Source: CAD feature listing. Evaluate the final solid. Frame: model axes, mm. Coordinates: 2 decimals unless noted, no trailing zeros. Order: outer loops, then holes, each group sorted by start corner. A loop starts at its lowest first (then second) coordinate and runs counter-clockwise, first axis right, second up. Notation, with made-up numbers: (43.5, -11.5) -> (76.5, -11.5) arc R30 cw to (76.5, 20.5) -> close; hole circle Ø5 at (75.25, 14.5). An arc over 180 degrees is marked (long way). Put each result on its own line as item: value.
from build123d import *

# Parameters (mm, degrees)
F1_DEPTH = 2
F2_R     = 5
F4_DEPTH = 2
F6_DEPTH = 2


# Not quite as in the source:
# - a feature names something its author has since deleted; it is built from what else it names


with BuildPart() as f1:
    # F0 (on Front) → F1 (new body)
    with BuildSketch(Plane.XZ):
        with BuildLine():
            Line((0, 5.5), (0, 0))
            Line((0, 0), (40, 0))
            Line((40, 0), (40, 5.5))
            Line((40, 5.5), (25, 5.5))
            ThreePointArc((25, 5.5), (22, 2.5), (19, 5.5))
            Line((19, 5.5), (0, 5.5))
        make_face()
        with BuildLine():
            Line((40, 5.5), (40, 0))
            Line((40, 0), (40, -2.5))
            ThreePointArc((40, -2.5), (41.05572809, 1.972135955), (44, 5.5))
            Line((44, 5.5), (40, 5.5))
        make_face()
        with BuildLine():
            Line((0, 11), (0, 5.5))
            Line((0, 5.5), (19, 5.5))
            ThreePointArc((19, 5.5), (22, 8.5), (25, 5.5))
            Line((25, 5.5), (40, 5.5))
            Line((40, 5.5), (40, 11))
            Line((40, 11), (0, 11))
        make_face()
        with BuildLine():
            Line((40, 11), (40, 5.5))
            Line((40, 5.5), (44, 5.5))
            ThreePointArc((44, 5.5), (41.05572809, 9.027864045), (40, 13.5))
            Line((40, 13.5), (40, 11))
        make_face()
        with BuildLine():
            Line((45, -2.5), (40, -2.5))
            ThreePointArc((40, -2.5), (50, -12.5), (60, -2.5))
            ThreePointArc((60, -2.5), (58.94427191, 1.972135955), (56, 5.5))
            ThreePointArc((56, 5.5), (53.1622776602, 4.0131670195), (50, 3.5))
            Line((50, 3.5), (50, 2.5))
            ThreePointArc((50, 2.5), (53.5355339059, 1.0355339059), (55, -2.5))
            ThreePointArc((55, -2.5), (50, -7.5), (45, -2.5))
        make_face()
        with BuildLine():
            ThreePointArc((44, 5.5), (41.05572809, 1.972135955), (40, -2.5))
            Line((40, -2.5), (45, -2.5))
            ThreePointArc((45, -2.5), (46.4644660941, 1.0355339059), (50, 2.5))
            Line((50, 2.5), (50, 3.5))
            ThreePointArc((50, 3.5), (46.8377223398, 4.0131670195), (44, 5.5))
        make_face()
        with BuildLine():
            ThreePointArc((40, 13.5), (41.05572809, 9.027864045), (44, 5.5))
            ThreePointArc((44, 5.5), (46.8377223398, 6.9868329805), (50, 7.5))
            Line((50, 7.5), (50, 8.5))
            ThreePointArc((50, 8.5), (46.4644660941, 9.9644660941), (45, 13.5))
            Line((45, 13.5), (40, 13.5))
        make_face()
        with BuildLine():
            Line((50, 5.5), (44, 5.5))
            ThreePointArc((44, 5.5), (46.8377223398, 4.0131670195), (50, 3.5))
            Line((50, 3.5), (50, 5.5))
        make_face()
        with BuildLine():
            ThreePointArc((50, 7.5), (46.8377223398, 6.9868329805), (44, 5.5))
            Line((44, 5.5), (50, 5.5))
            Line((50, 5.5), (50, 7.5))
        make_face()
        with BuildLine():
            ThreePointArc((60, 13.5), (50, 23.5), (40, 13.5))
            Line((40, 13.5), (45, 13.5))
            ThreePointArc((45, 13.5), (50, 18.5), (55, 13.5))
            ThreePointArc((55, 13.5), (53.5355339059, 9.9644660941), (50, 8.5))
            Line((50, 8.5), (50, 7.5))
            ThreePointArc((50, 7.5), (53.1622776602, 6.9868329805), (56, 5.5))
            ThreePointArc((56, 5.5), (58.94427191, 9.027864045), (60, 13.5))
        make_face()
        with BuildLine():
            ThreePointArc((56, 5.5), (53.1622776602, 6.9868329805), (50, 7.5))
            Line((50, 7.5), (50, 5.5))
            Line((50, 5.5), (56, 5.5))
        make_face()
        with BuildLine():
            Line((50, 5.5), (50, 3.5))
            ThreePointArc((50, 3.5), (53.1622776602, 4.0131670195), (56, 5.5))
            Line((56, 5.5), (50, 5.5))
        make_face()
    extrude(amount=F1_DEPTH)

    # F2
    f2_edges = [f1.edges().sort_by_distance(p)[0] for p in [
        (40, -1, 11),
        (40, -1, 0),
        (0, -1, 11),
        (0, -1, 0),
    ]]
    fillet(f2_edges, radius=F2_R)

    # F3 (on face) → F4 (cut, through all)
    with BuildSketch(Plane.XZ.offset(2)):
        with BuildLine():
            Line((19.0419601085, 6), (0, 6))
            Line((0, 6), (0, 5))
            Line((0, 5), (19.0419601085, 5))
            ThreePointArc((19.0419601085, 5), (19, 5.5), (19.0419601085, 6))
        make_face()
        with BuildLine():
            Line((30, 6), (24.9580398915, 6))
            ThreePointArc((24.9580398915, 6), (24.9894915684, 5.7508787808), (25, 5.5))
            ThreePointArc((25, 5.5), (24.9894915684, 5.2491212192), (24.9580398915, 5))
            Line((24.9580398915, 5), (30, 5))
            Line((30, 5), (30, 6))
        make_face()
    extrude(amount=-F4_DEPTH, mode=Mode.SUBTRACT)

    # F5 (on face) → F6 (join)
    with BuildSketch(Plane.XZ.offset(2)):
        with BuildLine():
            ThreePointArc((43.1634270419, -9.7980319394), (41.8309701191, -8.2677509312), (40.8348486101, -6.5))
            Line((40.8348486101, -6.5), (39.2329856296, -6.5))
            Line((39.2329856296, -6.5), (43.1634270419, -9.7980319394))
        make_face()
    extrude(amount=-F6_DEPTH)


solid = f1.part
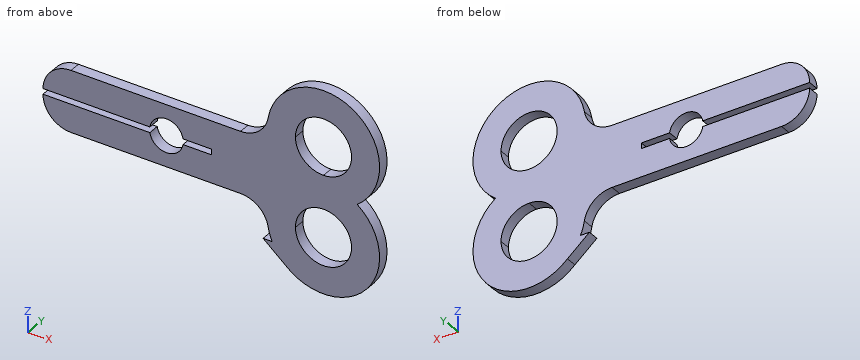
1. First-contact query: pin 1 (1 mm diameter, centred on y = -2, z = 18.5, fed in from -X); pin 2 (1 mm diameter, centred on x = 10.5, y = -0.5, fed in from +Z); pin 3 (1 mm diameter, centred on x = 15.5, y = -1, fed in from -Z); pin 4 (12 mm diameter, centred on x = 6.5, z = 19, fed in from +Y). Flat tips, straight axial feed; report the tip coordinate or a pass-through.
Numbers:
pin 1: stops at x = 41.07
pin 2: stops at z = 11
pin 3: stops at z = 0
pin 4: passes through
2. Cut plane C-C on x = 23.5. Output: boundary loops of the cut face in (y, z), plus the area to 3 significant figures.
Numbers:
outline: (-2, 0) -> (0, 0) -> (0, 2.9) -> (-2, 2.9) -> close; (-2, 8.1) -> (0, 8.1) -> (0, 11) -> (-2, 11) -> close
area: 11.6 mm2
3. Cut plane A-A on x = 54. Output: boundary loops of the cut face in (y, z), plus the area to 3 significant figures.
Numbers:
outline: (-2, -11.67) -> (0, -11.67) -> (0, -5.5) -> (-2, -5.5) -> close; (-2, 0.5) -> (0, 0.5) -> (0, 10.5) -> (-2, 10.5) -> close; (-2, 16.5) -> (0, 16.5) -> (0, 22.67) -> (-2, 22.67) -> close
area: 44.7 mm2
4. Cut plane D-D on y = -0.7. Count the separate pieces of the cut face and the enclosed holes in it, plus the area to 3 significant figures.
Numbers:
separate pieces: 1
enclosed holes: 2
area: 846 mm2
5. Ray query, line 1 along Z through (x, y) = (8, -0.25); line 2 along X through (y, z) = (-1.2, 11.5); line 3 along X through (y, z) = (-0.3, 10). Return the intervals inside material, ascending.
Numbers:
line 1: z = 0 to 5, 6 to 11
line 2: x = 37.39 to 45.42, 54.58 to 59.8
line 3: x = 2 to 46.43, 53.57 to 59.37
6. Cut plane B-B on z = 7. Output: boundary loops of the cut face in (x, y).
Numbers:
outline: (0.1, -2) -> (19.4, -2) -> (19.4, 0) -> (0.1, 0) -> close; (24.6, -2) -> (57.6, -2) -> (57.6, 0) -> (24.6, 0) -> close
